from build123d import *

# Parameters (mm, degrees)
SKETCH2_R                       = 21.59
SKETCH2_R_2                     = 17.145
BOSS_EXTRUDE1_DEPTH             = 83.82
BOSS_EXTRUDE1_DIRECTION_2_REACH = 111.985
SKETCH2_4_R                     = 17.145
CUT_EXTRUDE3_DEPTH              = 138.938
SKETCH4_R                       = 2.54
CUT_EXTRUDE4_DEPTH              = 138.938
CIRPATTERN1_COUNT               = 3


with BuildPart() as part:
    # Sketch1 → Revolve1 (revolve)
    with BuildSketch(Plane.XY):
        with BuildLine():
            Line((-63.5, 0), (-60.96, 0))
            ThreePointArc((-60.96, 0), (0, 60.96), (60.96, 0))
            Line((60.96, 0), (63.5, 0))
            ThreePointArc((63.5, 0), (0, 63.5), (-63.5, 0))
        make_face()
    revolve(axis=Axis((-63.5, 0, 0), (1, 0, 0)))

    # Sketch2 → Boss-Extrude1 (add)
    with BuildSketch(Plane(origin=(0, 0, 0), x_dir=(0, 0, -1), z_dir=(1, 0, 0))):
        with Locations((0, 10.0076)):
            Circle(SKETCH2_R)
        with Locations((0, 10.0076)):
            Circle(SKETCH2_R_2, mode=Mode.SUBTRACT)
    extrude(amount=BOSS_EXTRUDE1_DEPTH)

    # Sketch2 → Boss-Extrude1 direction 2 (add, up to next)
    with BuildSketch(Plane(origin=(0, 0, 0), x_dir=(0, 0, -1), z_dir=(1, 0, 0)), mode=Mode.PRIVATE) as boss_extrude1_direction_2_sk1:
        with Locations((0, 10.0076)):
            Circle(SKETCH2_R)
        with Locations((0, 10.0076)):
            Circle(SKETCH2_R_2, mode=Mode.SUBTRACT)
    boss_extrude1_direction_2_tool1 = extrude(boss_extrude1_direction_2_sk1.sketch, amount=-BOSS_EXTRUDE1_DIRECTION_2_REACH, mode=Mode.PRIVATE) - part.part
    add(boss_extrude1_direction_2_tool1.solids().sort_by_distance((0, 10.0076, 20.979343))[0])

    # Sketch2_4 → Cut-Extrude3 (cut)
    with BuildSketch(Plane(origin=(0, 0, 0), x_dir=(0, 0, -1), z_dir=(1, 0, 0))):
        with Locations((0, 10.0076)):
            Circle(SKETCH2_4_R)
    extrude(amount=CUT_EXTRUDE3_DEPTH, mode=Mode.SUBTRACT)

    # Sketch4 → Cut-Extrude4 (cut)
    with BuildSketch(Plane(origin=(0, 0, 0), x_dir=(1, 0, 0), z_dir=(0, 1, 0))):
        with Locations(Location((73.66, 0, 0), (0, 0, 270))):
            Circle(SKETCH4_R)
    cut_extrude4 = extrude(amount=-CUT_EXTRUDE4_DEPTH, mode=Mode.SUBTRACT)

    # CirPattern1: Cut-Extrude4 ×3 about axis
    cirpattern1_axis = Axis((-63.502, 10.0076, 0), (1, 0, 0))
    for i in range(1, CIRPATTERN1_COUNT):
        add(cut_extrude4.rotate(cirpattern1_axis, i * 360 / CIRPATTERN1_COUNT), mode=Mode.SUBTRACT)


solid = part.part
The listing builds one solid part. Answer for the finished solid, in the listing's coordinates (mm). A direction names the side the tool comes from. Give positions to 0.01 mm unless a question says otherwise; leave off trailing zeros. Write each loop counter-clockwise with the first axis right and the second up, starting at its lowest first coordinate (ties: lowest second). Pieces come first, ordered by that corner, then holes. Notation, with made-up numbers: (85, 67.5) - (142, 67.5) arc R23 ccw to (142, 89.5) - close; hole circle Ø8 at (19.5, 59.5). An arc over 180 degrees is marked (long way). Use a Markdown table: item, result.
1. Section A-A on z = 0 is taken. Write down the section's boundary in (x, y).
Values follow:
| item | result |
|---|---|
| outline | (-60.54, -7.14) arc R60.96 cw to (-54.58, 27.15) - (83.82, 27.15) - (83.82, 31.6) - (55.08, 31.6) arc R63.5 ccw (long way) to (62.43, -11.58) - (71.12, -11.58) - (71.12, -7.14) - close; (76.2, -11.58) - (83.82, -11.58) - (83.82, -7.14) - (76.2, -7.14) - close; hole (-59.85, -11.58) arc R60.96 ccw to (59.85, -11.58) - close; hole (-52.13, 31.6) - (52.13, 31.6) arc R60.96 ccw to start |
2. For a pull along Z with two mould halves and no side action, classify faces 4 (the cylindrical face through (71.18, 19.15, 16.94)), 5 (the flat face through (83.82, 28, -1)), 6 (the cylindrical face through (72.442, 31.414, 2.811)) as released by +Z, released by -Z, zero draft, split by the parting line, or undercut.
Values follow:
| item | result |
|---|---|
| face 4 | undercut |
| face 5 | zero draft |
| face 6 | split by the parting line |
3. Section B-B on x = 41.5 is taken. Write down the section's boundary in (y, z) (3 decimals).
Values follow:
| item | result |
|---|---|
| outline | circle Ø96.125 at (0, 0); circle Ø43.18 at (10.008, 0); hole circle Ø89.306 at (0, 0); hole circle Ø34.29 at (10.008, 0) |
4. Section D-D on x = 73.66 is taken. Write down the section's boundary in (y, z) (3 decimals).
Values follow:
| item | result |
|---|---|
| outline | (-11.432, -2.54) arc R21.59 ccw to (18.528, -19.838) - (16.286, -15.954) arc R17.145 cw to (-6.948, -2.54) - close; (-11.432, 2.54) - (-6.948, 2.54) arc R17.145 cw to (16.286, 15.954) - (18.528, 19.838) arc R21.59 ccw to start; (20.685, -13.414) - (22.927, -17.298) arc R21.59 ccw to (22.927, 17.298) - (20.685, 13.414) arc R17.145 cw to start |
5. Find the intervals of material crossed by probe 1 along Z at (x, y) = (-51.5, 10.5); probe 2 along Z at (x, y) = (5, 8.5); probe 3 along Y at (x, z) = (-28.5, 0), in increasing order. Write a range as from..to.
Values follow:
| item | result |
|---|---|
| probe 1 | z = -35.63..-30.88, -21.58..-17.14, 17.14..21.58, 30.88..35.63 |
| probe 2 | z = -62.73..-60.16, -21.54..-17.08, 17.08..21.54, 60.16..62.73 |
| probe 3 | y = -56.75..-53.89, -11.58..-7.14, 27.15..31.6, 53.89..56.75 |
6. A tool of negligible diameter and unlimited length cuts with its end or side. For faces 1 (the cylindrical face through (71.18, -9.23, -0.55)), 2 (the cylindrical face through (71.4, 18.6, -17.2)), 3 (the cylindrical face through (10.629, -5.203, -7.911)), from which of +Z, -Z, +X, -X, +Y, -Y can it reach the whole face along a straight path? Write none if from no direction.
Values follow:
| item | result |
|---|---|
| face 1 | -Y |
| face 2 | none |
| face 3 | +X |
7. Each of these flat-tipped pins is pushed along its axis until it touches: P1, Ø1.5, axis at y = -5.5, z = 6.5, coming from the -X side; P2, Ø4.5, axis at x = 73.66, z = 0, coming from the -Y side; P3, Ø1, axis at y = 1, z = -29.5, coming from the -X side. Where does it stop, or does it pass through?
Values follow:
| item | result |
|---|---|
| P1 | stops at x = -63.02 |
| P2 | stops at y = 27 |
| P3 | stops at x = -56.48 |
8. Section C-C on y = -4 is taken. Write down the section's boundary in (x, z), plus the area to 3 significant figures.
Values follow:
| item | result |
|---|---|
| outline | (-60.02, -9.89) arc R60.83 cw to (-60.02, 9.89) - (83.82, 9.89) - (83.82, 16.43) - (61.21, 16.43) arc R63.37 ccw (long way) to (61.21, -16.43) - (83.82, -16.43) - (83.82, -9.89) - close; hole (-58.57, -16.43) arc R60.83 ccw to (58.57, -16.43) - close; hole (-58.57, 16.43) - (58.57, 16.43) arc R60.83 ccw to start |
| area | 2,780 mm² |
